from build123d import *

# Parameters (mm, degrees)
SKETCH2_W           = 1.66
SKETCH2_H           = 30.07
SKETCH3_R           = 1.225
CUT_EXTRUDE1_DEPTH  = 2.66
SKETCH3_3_R         = 3.175
SKETCH3_3_R_2       = 1.225
BOSS_EXTRUDE1_DEPTH = 1.43


with BuildPart() as part:
    # Sweep1: sweep along a path in Sketch1
    with BuildLine(Plane(origin=(0, 0, 0), x_dir=(1, 0, 0), z_dir=(0, 1, 0))) as sweep1_path:
        Line((-45.14, 0), (-30.89, 0))
        ThreePointArc((-30.89, 0), (-30.182893219, 0.292893219), (-29.89, 1))
        Line((-29.89, 1), (-29.89, 31.63))
        ThreePointArc((-29.89, 31.63), (-29.597106781, 32.337106781), (-28.89, 32.63))
        Line((-28.89, 32.63), (28.89, 32.63))
        ThreePointArc((28.89, 32.63), (29.597106781, 32.337106781), (29.89, 31.63))
        Line((29.89, 31.63), (29.89, 1))
        ThreePointArc((29.89, 1), (30.182893219, 0.292893219), (30.89, 0))
        Line((30.89, 0), (45.14, 0))
    # Sketch2 → Sweep1 (sweep)
    with BuildSketch(Plane(origin=(45.14, 0, 0), x_dir=(0, 0, -1), z_dir=(1, 0, 0))):
        Rectangle(SKETCH2_W, SKETCH2_H)
    sweep(path=sweep1_path.line)

    # Sketch3 → Cut-Extrude1 (cut, through all)
    with BuildSketch(Plane(origin=(0, 0, -0.83), x_dir=(-1, 0, 0), z_dir=(0, 0, -1))):
        with Locations((-34.5, 0)):
            Circle(SKETCH3_R)
    cut_extrude1 = extrude(amount=-CUT_EXTRUDE1_DEPTH, mode=Mode.SUBTRACT)

    # Sketch3_3 → Boss-Extrude1 (add)
    with BuildSketch(Plane(origin=(0, 0, -0.83), x_dir=(-1, 0, 0), z_dir=(0, 0, -1))):
        with Locations((-34.5, 0)):
            Circle(SKETCH3_3_R)
        with Locations((-34.5, 0)):
            Circle(SKETCH3_3_R_2, mode=Mode.SUBTRACT)
    boss_extrude1 = extrude(amount=BOSS_EXTRUDE1_DEPTH)

    # Mirror1: Cut-Extrude1, Boss-Extrude1 across plane
    add(cut_extrude1.mirror(Plane(origin=(0, 0, 0), x_dir=(0, 0, 1), z_dir=(1, 0, 0))), mode=Mode.SUBTRACT)
    add(boss_extrude1.mirror(Plane(origin=(0, 0, 0), x_dir=(0, 0, 1), z_dir=(1, 0, 0))))


solid = part.part
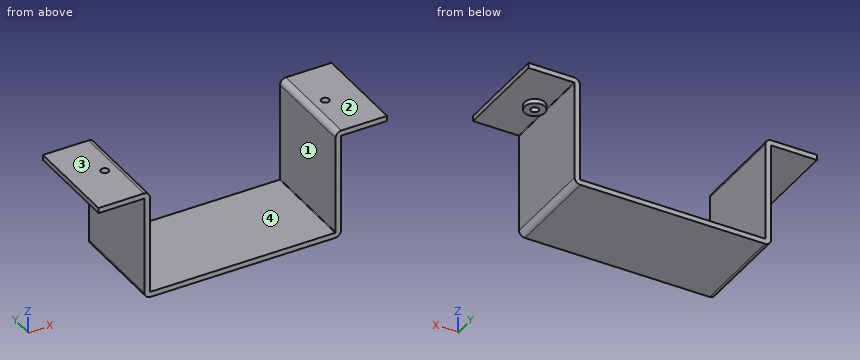
The model under review builds one solid part; all positions refer to its coordinate system, in mm. Face numbers are marked on the shaded views. A direction names the side the tool comes from. Round coordinates to 2 decimals unless told otherwise and drop trailing zeros. Loops run counter-clockwise (first coordinate to the right, second up) from the corner with the lowest first, then second, coordinate; pieces in that order, holes last. Notation, with made-up numbers: (71.5, -30) - (77.5, -30) arc R17 ccw to (77.5, -13) - close; hole circle Ø9 at (5, 45.25). An arc over 180 degrees is marked (long way). Use CSV: the item, a comma, the result in double quotes.
(1) Machinability: for the marked faces 1 and 2, which of the approach directions +Z, -Z, +X, -X, +Y, -Y give a long, thin tool a straight path to every point of the face, cutting with its end or side? Answer none if there is none.
Working result:
face 1,"+Z, +Y, -Y"
face 2,"+Z, +X, -X, +Y, -Y"
(2) Take a section at A-A, the plane x = 34.5. Give the boundary of the cut face in (y, z) (3 decimals), plus the area to 3 significant figures.
Working result:
outline,"(-15.035, -0.83) - (-3.175, -0.83) - (-3.175, -2.26) - (-1.225, -2.26) - (-1.225, 0.83) - (-15.035, 0.83) - close; (1.225, -2.26) - (3.175, -2.26) - (3.175, -0.83) - (15.035, -0.83) - (15.035, 0.83) - (1.225, 0.83) - close"
area,"51.4 mm^2"
(3) Take a section at D-D, the plane y = 0. State how many separate pieces and enclosed holes the cut face has, plus the area to 3 significant figures.
Working result:
separate pieces,"3"
enclosed holes,"0"
area,"258 mm^2"
(4) The part is to be moulded in two halves that separate along X. For the marked faces 3 and 4, say which applies: pulls with the +X half, pulls with the -X half, needs draft (parallel to the pull), parting line crosses it, or undercut.
Working result:
face 3,"needs draft"
face 4,"undercut"
(5) Take a section at B-B, the plane z = -29.5. Give the boundary of the cut face in (x, y) (3 decimals).
Working result:
outline,"(-30.72, -15.035) - (-29.06, -15.035) - (-29.06, 15.035) - (-30.72, 15.035) - close; (29.06, -15.035) - (30.72, -15.035) - (30.72, 15.035) - (29.06, 15.035) - close"
(6) Clearance check with flat-ended pins moving along their axes: P1, Ø9, axis at y = -5.5, z = -18.5, coming from the +X side; P2, Ø5, axis at x = 33, y = 0, coming from the -Z side; P3, Ø1.5, axis at y = 9.5, z = -4.5, coming from the -X side; P4, Ø6, axis at x = 25.5, z = -26.5, coming from the +Y side. State where each tip first meets the part, or that it passes through.
Working result:
P1,"stops at x = 30.72"
P2,"stops at z = -32.5"
P3,"stops at x = -30.72"
P4,"passes through"
(7) Take a section at C-C, the plane y = -4.5. Give the boundary of the cut face in (x, z).
Working result:
outline,"(-45.14, -0.83) - (-30.89, -0.83) arc R0.17 cw to (-30.72, -1) - (-30.72, -31.63) arc R1.83 ccw to (-28.89, -33.46) - (28.89, -33.46) arc R1.83 ccw to (30.72, -31.63) - (30.72, -1) arc R0.17 cw to (30.89, -0.83) - (45.14, -0.83) - (45.14, 0.83) - (30.89, 0.83) arc R1.83 ccw to (29.06, -1) - (29.06, -31.63) arc R0.17 cw to (28.89, -31.8) - (-28.89, -31.8) arc R0.17 cw to (-29.06, -31.63) - (-29.06, -1) arc R1.83 ccw to (-30.89, 0.83) - (-45.14, 0.83) - close"
(8) For line 1 (X direction, y = 12, z = -2.5); line 2 (Y direction, x = -34.5, z = -0.9) (3 decimals); line 3 (Z direction, x = -8, y = -11), list the stretches that pass through material, from the lowest coordinate up.
Working result:
line 1,"x = -30.72 to -29.06, 29.06 to 30.72"
line 2,"y = -3.175 to -1.225, 1.225 to 3.175"
line 3,"z = -33.46 to -31.8"
